```python
from build123d import *

# Parameters (mm, degrees)
BOSS_EXTRUDE1_DEPTH = 239
SKETCH2_R           = 1.599999999999998
SKETCH2_R_2         = 1.5999999999999908
CUT_EXTRUDE1_DEPTH  = 240.44586691023747
BOSS_EXTRUDE2_DEPTH = 1.6
FILLET1_R           = 2
SKETCH4_W           = 302.77939153503445
SKETCH4_H           = 48.73306397089993
CUT_EXTRUDE2_DEPTH  = 0.55


with BuildPart() as part:
    # Sketch1 → Boss-Extrude1 (new body)
    with BuildSketch(Plane(origin=(0, 0, 0), x_dir=(0, 0, -1), z_dir=(1, 0, 0))):
        Polygon((2.5431313581277277, 8.378511762801937), (-0.1315705594718698, 1.029828640425271), (-8.118957836152065, 3.936999858693529), (-4.86976647455813, 12.864079756159628), (3.117620802122064, 9.95690853789137), align=None)
    extrude(amount=BOSS_EXTRUDE1_DEPTH)

    # Sketch2 → Cut-Extrude1 (cut, through all)
    with BuildSketch(Plane(origin=(0, 9.794155508645982, -3.5647810749215956), x_dir=(1, 0, 0), z_dir=(0, 0.9396926207859053, -0.3420201433256773))):
        with Locations(Location((5.999999999999991, -4.047641310446752, 0), (0, 0, 270))):
            Circle(SKETCH2_R)
        with Locations(Location((232.99999999999997, -4.047641310446725, 0), (0, 0, 270))):
            Circle(SKETCH2_R_2)
    extrude(amount=-CUT_EXTRUDE1_DEPTH, mode=Mode.SUBTRACT)

    # Sketch3 → Boss-Extrude2 (add)
    with BuildSketch(Plane(origin=(0, 0.8670756111798825, -0.31558971332766134), x_dir=(1, 0, 0), z_dir=(0, 0.9396926207859052, -0.34202014332567726))):
        Polygon((0, -0.47585802304752833), (1.5, -0.47585802304752783), (1.5000000000000013, -8.975858023047525), (0, -8.975858023047529), align=None)
        Polygon((239, -0.47585802304752833), (237.5, -0.475858023047528), (237.5, -8.975858023047525), (239, -8.975858023047529), align=None)
    extrude(amount=-BOSS_EXTRUDE2_DEPTH)

    # Fillet1
    fillet1_edges = [part.edges().sort_by_distance(p)[0] for p in [
        (239, 7.6487857107978545, 6.76797827001564),
        (0, 7.648785710797854, 6.76797827001564),
    ]]
    fillet(fillet1_edges, radius=FILLET1_R)

    # Sketch4 → Cut-Extrude2 (cut)
    with BuildSketch(Plane(origin=(0, 9.794155508645986, -3.5647810749215965), x_dir=(1, 0, 0), z_dir=(0, 0.9396926207859053, -0.34202014332567743))):
        with Locations((120.43717430713222, 0.7530071571181338)):
            Rectangle(SKETCH4_W, SKETCH4_H)
    extrude(amount=-CUT_EXTRUDE2_DEPTH, mode=Mode.SUBTRACT)


solid = part.part
```
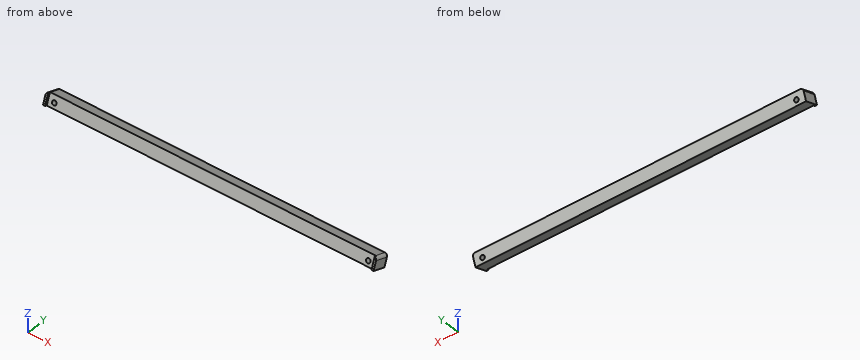
For this review, take the finished solid that the model builds, in its own axes (mm). Give positions to 0.01 mm unless a question says otherwise; leave off trailing zeros. Loops run counter-clockwise (first coordinate to the right, second up) from the corner with the lowest first, then second, coordinate; pieces in that order, holes last. Notation, with made-up numbers: M 70,-28 L 122,-28 A25 ccw 122,-3 Z; hole C 11.5,9 d5. An arc over 180 degrees is marked long. One line per item, written item: value. Start each with the question number.
Q1. For L1, parallel to X at y = 10, z = 4.25; L2, parallel to X at y = 0.5, z = 3; L3, parallel to Y at x = 78.5, z = 2, list the stretches that pass through material, from the lowest coordinate up.
Q2. Add section B-B (y = 6.5). Count the separate pieces of the cut face and the enclosed holes in it, and give its area (3 significant figures).
Q3. Clearance check with flat-ended pins moving along their axes: pin 1 Ø4 at (x, z) = (39, 0) entering from +Y; pin 2 Ø1.5 at (x, z) = (75.5, 0.5) entering from +Y; pin 3 Ø2 at (x, y) = (140, 9) entering from -Z. State where each tip first meets the part, or that it passes through.
Q4. Add section A-A (x = 89.5). Give the boundary of the cut face in (y, z).
Reply:
1. L1: 0.05 to 238.95
1. L2: 0 to 1.5, 237.5 to 239
1. L3: 1.71 to 11.23
2. separate pieces: 1
2. enclosed holes: 2
2. area: 2,140 mm²
3. pin 1: y = 11.23
3. pin 2: y = 10.96
3. pin 3: z = -2.93
4. outline: M 1.03,0.13 L 9.44,-2.93 L 12.35,5.06 L 3.94,8.12 Z
